from build123d import *

# Parameters (mm, degrees)
ESQUISSE1_W             = 20
ESQUISSE1_H             = 20
BOSS_EXTRU_1_DEPTH      = 24
BOSS_EXTRU_2_DEPTH      = 25
BOSS_EXTRU_3_DEPTH      = 25
BOSS_EXTRU_4_DEPTH      = 25
BOSS_EXTRU_5_DEPTH      = 25
ESQUISSE6_R             = 3
ENL_V_MAT_EXTRU_1_DEPTH = 22


with BuildPart() as part:
    # Esquisse1 → Boss.-Extru.1 (new body)
    with BuildSketch(Plane.XY):
        Rectangle(ESQUISSE1_W, ESQUISSE1_H)
    extrude(amount=BOSS_EXTRU_1_DEPTH)

    # Esquisse2 → Boss.-Extru.2 (add)
    with BuildSketch(Plane.XY.offset(24)):
        Polygon((-2.45, -10), (-2.45, -8.45), (-6.15, -8.45), (-6.15, -7.45), (-2.645559959, -3.8), (2.654440041, -3.8), (6.15, -7.458505237), (6.15, -8.45), (2.45, -8.45), (2.45, -10), align=None)
    extrude(amount=BOSS_EXTRU_2_DEPTH)

    # Esquisse3 → Boss.-Extru.3 (add)
    with BuildSketch(Plane.XY.offset(24)):
        Polygon((10, -2.45), (8.45, -2.45), (8.45, -6.15), (7.45, -6.15), (3.8, -2.645559959), (3.8, 2.654440041), (7.45, 6.15), (8.45, 6.15), (8.45, 2.45), (10, 2.45), align=None)
    extrude(amount=BOSS_EXTRU_3_DEPTH)

    # Esquisse4 → Boss.-Extru.4 (add)
    with BuildSketch(Plane.XY.offset(24)):
        Polygon((2.45, 10), (2.45, 8.45), (6.15, 8.45), (6.15, 7.45), (2.645559959, 3.8), (-2.654440041, 3.8), (-6.15, 7.458505237), (-6.15, 8.45), (-2.45, 8.45), (-2.45, 10), align=None)
    extrude(amount=BOSS_EXTRU_4_DEPTH)

    # Esquisse5 → Boss.-Extru.5 (add)
    with BuildSketch(Plane.XY.offset(24)):
        Polygon((-10, 2.45), (-8.45, 2.45), (-8.45, 6.15), (-7.45, 6.15), (-3.8, 2.645559959), (-3.8, -2.654440041), (-7.45, -6.15), (-8.45, -6.15), (-8.45, -2.45), (-10, -2.45), align=None)
    extrude(amount=BOSS_EXTRU_5_DEPTH)

    # Esquisse6 → Enlèv. mat.-Extru.1 (cut)
    with BuildSketch(Plane(origin=(0, 0, 0), x_dir=(-1, 0, 0), z_dir=(0, 0, -1))):
        Circle(ESQUISSE6_R)
    extrude(amount=-ENL_V_MAT_EXTRU_1_DEPTH, mode=Mode.SUBTRACT)


solid = part.part
Geometry check sheet. Reference: the model listing, model coordinates, mm. A direction names the side the tool comes from. Give positions to 0.01 mm unless a question says otherwise; leave off trailing zeros. Loops run counter-clockwise (first coordinate to the right, second up) from the corner with the lowest first, then second, coordinate; pieces in that order, holes last. Notation, with made-up numbers: (27, -35) -> (61, -35) arc R34 ccw to (61, 3) -> close; hole circle Ø5 at (23.25, -16.5). An arc over 180 degrees is marked (long way). Answer in a Markdown table with one row per item. Add a question column.
1) Cross-section at C-C on z = 20.5. Record the boundary of the cut face in (x, y).
2) Set-up check for faces 1 (the face through (-4, 8.45, 36)), 2 (the face through (4.42, 5.65, 36.33)), 3 (the face through (2.45, 9, 36)), 4 (the face through (-9, -2.45, 36)): record each of +Z, -Z, +X, -X, +Y, -Y from which the full face is reachable in a straight line by a thin tool's end or side.
3) Gauge pin test, flat ends, axial feed: P1, Ø0.5, axis at y = 9.5, z = 37, coming from the +X side; P2, Ø0.8, axis at y = 9.5, z = 36.5, coming from the -X side; P3, Ø1.7, axis at x = 9.5, z = 40, coming from the +Y side. Record the tip position at first contact, or that the pin passes through.
4) Material ranges on probe 1 along Y at (x, z) = (0, 17); probe 2 along X at (y, z) = (0.75, 43); probe 3 along X at (y, z) = (-4.25, 39), recorded low to high. Write a range as from..to.
5) Cross-section at A-A on y = 0. Record the boundary of the cut face in (x, z), and give its area (3 significant figures).
6) Cross-section at D-D on z = 40. State how many separate pieces and enclosed holes the cut face has, and give its area (3 significant figures).
7) Draft check along X on faces 5 (the face through (-2.45, 9, 36)), 6 (the face through (4, -8.45, 36)), 7 (the face through (6.15, 8, 36)), 8 (the face through (5.6, 4.38, 36.33)). Enter one of: pulls with the +X half, pulls with the -X half, needs draft (parallel to the pull), parting line crosses it, or undercut.
Outcome:
| question | item | result |
|---|---|---|
| 1 | outline | (-10, -10) -> (10, -10) -> (10, 10) -> (-10, 10) -> close; hole circle Ø6 at (0, 0) |
| 2 | face 1 | +Z, -X, +Y |
| 2 | face 2 | +Z |
| 2 | face 3 | +Z, +X, +Y |
| 2 | face 4 | +Z, -X, -Y |
| 3 | P1 | stops at x = 2.45 |
| 3 | P2 | stops at x = -2.45 |
| 3 | P3 | stops at y = 2.45 |
| 4 | probe 1 | y = -10..-3, 3..10 |
| 4 | probe 2 | x = -10..-3.8, 3.8..10 |
| 4 | probe 3 | x = -8.45..-5.47, -3.08..3.08, 5.47..8.45 |
| 5 | outline | (-10, 0) -> (-3, 0) -> (-3, 22) -> (3, 22) -> (3, 0) -> (10, 0) -> (10, 49) -> (3.8, 49) -> (3.8, 24) -> (-3.8, 24) -> (-3.8, 49) -> (-10, 49) -> close |
| 5 | area | 658 mm^2 |
| 6 | separate pieces | 4 |
| 6 | enclosed holes | 0 |
| 6 | area | 208 mm^2 |
| 7 | face 5 | pulls with the -X half |
| 7 | face 6 | needs draft |
| 7 | face 7 | pulls with the +X half |
| 7 | face 8 | undercut |
